from build123d import *

# Parameters (mm, degrees)
ESBO_O1_R                = 1.5
ESBO_O1_R_2              = 3.65
RESSALTO_EXTRUS_O1_DEPTH = 5
CORTE_EXTRUS_O1_DEPTH    = 3


with BuildPart() as part:
    # Esbo_o1 → Ressalto-extrus_o1 (new body)
    with BuildSketch(Plane.XY):
        with BuildLine():
            Line((-6, 2), (-6, -24))
            Line((-6, -24), (2, -32))
            Line((2, -32), (20, -32))
            Line((20, -32), (20, -24))
            Line((20, -24), (6, -24))
            Line((6, -24), (6, 2))
            ThreePointArc((6, 2), (4.828427125, 4.828427125), (2, 6))
            Line((2, 6), (-2, 6))
            ThreePointArc((-2, 6), (-4.828427125, 4.828427125), (-6, 2))
        make_face()
        with Locations((5.5, -28)):
            Circle(ESBO_O1_R, mode=Mode.SUBTRACT)
        Circle(ESBO_O1_R_2, mode=Mode.SUBTRACT)
        with BuildLine():
            Line((-0.7, -14.5), (-0.7, -11.5))
            ThreePointArc((-0.7, -11.5), (0, -10.8), (0.7, -11.5))
            Line((0.7, -11.5), (0.7, -14.5))
            ThreePointArc((0.7, -14.5), (0, -15.2), (-0.7, -14.5))
        make_face(mode=Mode.SUBTRACT)
        with BuildLine():
            Line((16.5, -26.5), (14.5, -26.5))
            ThreePointArc((14.5, -26.5), (13, -28), (14.5, -29.5))
            Line((14.5, -29.5), (16.5, -29.5))
            ThreePointArc((16.5, -29.5), (18, -28), (16.5, -26.5))
        make_face(mode=Mode.SUBTRACT)
    extrude(amount=RESSALTO_EXTRUS_O1_DEPTH)

    # Esbo_o1_3 → Corte-extrus_o1 (cut)
    with BuildSketch(Plane.XY):
        with BuildLine():
            ThreePointArc((-2.238721733, -14.225), (0, -16.25), (2.238721733, -14.225))
            Line((2.238721733, -14.225), (3.631704145, -0.365))
            ThreePointArc((3.631704145, -0.365), (0, -3.65), (-3.631704145, -0.365))
            Line((-3.631704145, -0.365), (-2.238721733, -14.225))
        make_face()
        with BuildLine():
            ThreePointArc((0.7, -14.5), (0, -15.2), (-0.7, -14.5))
            Line((-0.7, -14.5), (-0.7, -11.5))
            ThreePointArc((-0.7, -11.5), (0, -10.8), (0.7, -11.5))
            Line((0.7, -11.5), (0.7, -14.5))
        make_face(mode=Mode.SUBTRACT)
    extrude(amount=CORTE_EXTRUS_O1_DEPTH, mode=Mode.SUBTRACT)


solid = part.part
Here's how the part is built. I have some questions about the finished solid (model axes, mm). A direction names the side the tool comes from. Coordinates: 2 decimals unless noted, no trailing zeros. Order: outer loops, then holes, each group sorted by start corner. A loop starts at its lowest first (then second) coordinate and runs counter-clockwise, first axis right, second up. Notation, with made-up numbers: (-22.5, 28.5) - (-16.5, 28.5) arc R7 ccw to (-16.5, 35.5) - close; hole circle Ø7 at (24, -11.75). An arc over 180 degrees is marked (long way). Use CSV: the item, a comma, the result in double quotes. Start each with the question number.
1. Suppose I cut it at D-D on y = -1.5. List the corners of the cut face in (x, z) for me, then the cut area to 3 significant figures.
2. For faces 5 (the face through (0.7, -13, 4)), 6 (the face through (-6, -11, 2)), 7 (the face through (13, -24, 2)), 8 (the face through (-0.05, -16.25, 1.48)), 9 (the face through (-2, -28, 2)), which set-ups out of +Z, -Z, +X, -X, +Y, -Y let a thin tool reach every point of the face, with its end or its side?
3. If we mould it in two halves opening along Y, with no side actions, what happens to faces 1 (the face through (20, -28, 2)), 2 (the face through (-2.945, -7.198, 1.479)), 3 (the face through (-4.797, 4.859, 2.465)), 4 (the face through (15, -29.5, 2))? For each: +Y half, -Y half, draft (parallel to the pull), parting line (faces both ways), or undercut.
4. I'm going to push flat-ended pins straight in: pin 1 (1.5 mm diameter, centred on x = 0.5, z = 0.5, fed in from -Y); pin 2 (1.6 mm diameter, centred on x = 15, z = 3, fed in from +Y); pin 3 (0.6 mm diameter, centred on y = -12.5, z = 4, fed in from +X). Where does each tip first touch, or does it pass through?
5. Suppose I cut it at C-C on x = 0. List the corners of the cut face in (y, z) for me, then the cut area to 3 significant figures.
6. Please list where these lines run through material, in increasing order: line 1 (X direction, y = 0, z = 3.8); line 2 (X direction, y = -29, z = 3.5); line 3 (X direction, y = -12.5, z = 3.25). Write a range as from..to.
7. Suppose I cut it at A-A on z = 0.5. List the corners of the cut face in (x, y) for me (3 decimals).
8. Suppose I cut it at B-B on y = -28. List the corners of the cut face in (x, z) for me.
Output:
1,outline,"(-6, 0) - (-3.52, 0) - (-3.52, 3) - (-3.33, 3) - (-3.33, 5) - (-6, 5) - close; (3.33, 3) - (3.52, 3) - (3.52, 0) - (6, 0) - (6, 5) - (3.33, 5) - close"
1,area,"25.6 mm2"
2,face 5,"+Z, -Z"
2,face 6,"+Z, -Z, -X, +Y, -Y"
2,face 7,"+Z, -Z, +X, +Y"
2,face 8,"-Z"
2,face 9,"+Z, -Z, -X, -Y"
3,face 1,"draft"
3,face 2,"undercut"
3,face 3,"+Y half"
3,face 4,"undercut"
4,pin 1,"stops at y = -31.25"
4,pin 2,"stops at y = -24"
4,pin 3,"stops at x = 6"
5,outline,"(-30, 0) - (-16.25, 0) - (-16.25, 3) - (-15.2, 3) - (-15.2, 5) - (-30, 5) - close; (-10.8, 3) - (-3.65, 3) - (-3.65, 5) - (-10.8, 5) - close; (3.65, 0) - (6, 0) - (6, 5) - (3.65, 5) - close"
5,area,"96.9 mm2"
6,line 1,"x = -6..-3.65, 3.65..6"
6,line 2,"x = -1..4.38, 6.62..13.38, 17.62..20"
6,line 3,"x = -6..-0.7, 0.7..6"
7,outline,"(-6, -24) - (2, -32) - (20, -32) - (20, -24) - (6, -24) - (6, 2) arc R4 ccw to (2, 6) - (-2, 6) arc R4 ccw to (-6, 2) - close; hole (-3.632, -0.365) - (-2.239, -14.225) arc R2.25 ccw to (2.239, -14.225) - (3.632, -0.365) arc R3.65 ccw (long way) to start; hole circle Ø3 at (5.5, -28); hole (14.5, -29.5) - (16.5, -29.5) arc R1.5 ccw to (16.5, -26.5) - (14.5, -26.5) arc R1.5 ccw to start"
8,outline,"(-2, 0) - (4, 0) - (4, 5) - (-2, 5) - close; (7, 0) - (13, 0) - (13, 5) - (7, 5) - close; (18, 0) - (20, 0) - (20, 5) - (18, 5) - close"
